Can you work these out from the model? Positions are in its coordinate system, mm. A direction names the side the tool comes from. Coordinates: 2 decimals unless noted, no trailing zeros. Write each loop counter-clockwise with the first axis right and the second up, starting at its lowest first coordinate (ties: lowest second). Pieces come first, ordered by that corner, then holes. Notation, with made-up numbers: (9, 26) - (55, 26) arc R16 ccw to (55, 55) - close; hole circle Ø5 at (41.5, -6). An arc over 180 degrees is marked (long way). Use one line per item in the form item = value. Start each with the question number.
(1) For pin 1 Ø5 at (x, y) = (52, 20.5) entering from -Z; pin 2 Ø5.5 at (x, z) = (50, -32) entering from +Y; pin 3 Ø5 at (x, z) = (54, -9.5) entering from +Y, each with a flat end and sliding along its axis, tell me the tip position at first contact or that it passes through.
(2) If we section it at B-B on z = -4: Please give me the cut outline in (x, y), then the cut area to 3 significant figures.
(3) On a 3-axis mill with a long thin cutter (end or side, diameter ignored), from which of +Z, -Z, +X, -X, +Y, -Y can I reach the whole of each face in a straight line? I mean faces 1 (the face through (37, 9, -35.206)), 2 (the face through (9.7, 4.7, 32.1)), 3 (the face through (5.601, 10.229, -23.467)). Say none if no direction works.
(4) If we section it at D-D on x = 27.5: Please give me the cut outline in (y, z), then the cut area to 3 significant figures.
(5) If we section it at C-C on y = 9: Please give me the cut outline in (x, z).
(6) If I drill on probe 1 along Z at (x, y) = (70.5, 11.25); probe 2 along Y at (x, z) = (67, 24); probe 3 along Y at (x, z) = (32, 8.5), over which ranges is the centre line in solid material (lowest first)? Write a range as from..to.
(7) Thinking about a two-plate mould opening in Z: for faces 4 (the face through (50.05, 5.16, 31.76)), 5 (the face through (36.98, 5.78, -4.37)), 6 (the face through (71.686, 10.229, -24.311)), 7 (the face through (75, 12, -7)), which applies, pulls with the +Z half, pulls with the -Z half, needs draft (parallel to the pull), parting line crosses it, or undercut?
(8) If we section it at A-A on x = 5: Please give me the cut outline in (y, z).
```python
from build123d import *

# Parameters (mm, degrees)
BOSS_EXTRUDE1_DEPTH = 75
SKETCH2_R           = 2
CUT_EXTRUDE1_DEPTH  = 10
CUT_EXTRUDE2_DEPTH  = 10
SKETCH3_R           = 2.543008444
CUT_EXTRUDE3_DEPTH  = 100
CHAMFER1_SIZE       = 2


with BuildPart() as part:
    # Sketch1 → Boss-Extrude1 (new body)
    with BuildSketch(Plane(origin=(0, 0, 0), x_dir=(0, 0, -1), z_dir=(1, 0, 0))):
        Polygon((-35.447605249, 4.173188871), (35.206481481, 4.173188871), (35.206481481, 14.173188871), (24.552394751, 14.173188871), (8.571096195, 24.699446456), align=None)
    extrude(amount=BOSS_EXTRUDE1_DEPTH)

    # Sketch2 → Cut-Extrude1 (cut)
    with BuildSketch(Plane(origin=(0, 14.173188871, 0), x_dir=(1, 0, 0), z_dir=(0, 1, 0))):
        with Locations(Location((5, 25.374559272, 0), (0, 0, 270))):
            Circle(SKETCH2_R)
        with Locations(Location((69.999998904, 25.386498054, 0), (0, 0, 270))):
            Circle(SKETCH2_R)
    extrude(amount=-CUT_EXTRUDE1_DEPTH, mode=Mode.SUBTRACT)

    # Sketch4 → Cut-Extrude2 (cut)
    with BuildSketch(Plane(origin=(0, 17.005051997, 7.929585973), x_dir=(1, 0, 0), z_dir=(0, 0.9063077870366527, 0.42261826174069383))):
        Polygon((0, -30.362774842), (7.065850082, -25.103103439), (13.976560291, -30.362774842), align=None)
        Polygon((22.065850082, -25.103103439), (28.976560291, -30.362774842), (15, -30.362774842), align=None)
        Polygon((37.065850082, -25.103103439), (43.976560291, -30.362774842), (30, -30.362774842), align=None)
        Polygon((52.065850082, -25.103103439), (58.976560291, -30.362774842), (45, -30.362774842), align=None)
        Polygon((67.065850082, -25.103103439), (73.976560291, -30.362774842), (60, -30.362774842), align=None)
    extrude(amount=-CUT_EXTRUDE2_DEPTH, mode=Mode.SUBTRACT)

    # Sketch3 → Cut-Extrude3 (cut)
    with BuildSketch(Plane.ZY):
        with Locations((-5.547587106, 8.033515635)):
            Circle(SKETCH3_R)
    extrude(amount=-CUT_EXTRUDE3_DEPTH, mode=Mode.SUBTRACT)

    # Chamfer1
    chamfer1_edges = [part.edges().sort_by_distance(p)[0] for p in [
        (5, 4.173188871, -27.374559272),
        (69.999998904, 4.173188871, -27.386498054),
    ]]
    chamfer(chamfer1_edges, length=CHAMFER1_SIZE)


solid = part.part
```
Reported:
q1.pin_1 = -18.74
q1.pin_2 = 14.17
q1.pin_3 = 24.7
q2.outline = (0, 4.17) - (75, 4.17) - (75, 6.02) - (0, 6.02) - close; (0, 10.05) - (75, 10.05) - (75, 22.57) - (0, 22.57) - close
q2.area = 1,080 mm2
q3.face_1 = -Z, +X, -X, +Y, -Y
q3.face_2 = +Z, -Y
q3.face_3 = -Y
q4.outline = (4.17, -35.21) - (14.17, -35.21) - (14.17, -24.55) - (24.7, -8.57) - (4.65, 34.43) - (4.17, 34.21) - close; hole circle Ø5.09 at (8.03, -5.55)
q4.area = 782 mm2
q5.outline = (0, -35.21) - (75, -35.21) - (75, -7.9) - (0, -7.9) - close; (0, -3.2) - (75, -3.2) - (75, 25.1) - (0, 25.1) - close; hole circle Ø4 at (5, -25.37); hole circle Ø4 at (70, -25.39)
q6.probe_1 = -35.21..-27.32, -23.45..20.27
q6.probe_2 = 4.17..9.51
q6.probe_3 = 4.17..16.74
q7.face_4 = pulls with the +Z half
q7.face_5 = undercut
q7.face_6 = undercut
q7.face_7 = needs draft
q8.outline = (4.17, -35.21) - (14.17, -35.21) - (14.17, -27.37) - (6.17, -27.37) - (4.17, -29.37) - close; (4.17, -21.37) - (6.17, -23.37) - (14.17, -23.37) - (14.17, -24.55) - (24.7, -8.57) - (5.75, 32.07) - (4.17, 31.34) - close; hole circle Ø5.09 at (8.03, -5.55)
